```python
from build123d import *

# Parameters (mm, degrees)
SKETCH3_R           = 2.25
SKETCH3_W           = 78.47813411
SKETCH3_H           = 26
BOSS_EXTRUDE1_DEPTH = 3
SKETCH4_W           = 86.47813411
SKETCH4_H           = 3
BOSS_EXTRUDE2_DEPTH = 10


with BuildPart() as part:
    # Sketch3 → Boss-Extrude1 (new body)
    with BuildSketch(Plane(origin=(0, 0, 0), x_dir=(1, 0, 0), z_dir=(0, 1, 0))):
        Polygon((-43.239067055, -30), (-43.239067055, 30), (-39.239067055, 30), (-39.239067055, 21), (39.239067055, 21), (39.239067055, 30), (43.239067055, 30), (43.239067055, -30), (39.239067055, -30), (39.239067055, -21), (-39.239067055, -21), (-39.239067055, -30), align=None)
        with Locations(Location((-26.009067055, 17, 0), (0, 0, 270))):
            Circle(SKETCH3_R, mode=Mode.SUBTRACT)
        with Locations(Location((3.760932945, 16.578763023, 0), (0, 0, 270))):
            Circle(SKETCH3_R, mode=Mode.SUBTRACT)
        with Locations(Location((26.009067055, 17, 0), (0, 0, 270))):
            Circle(SKETCH3_R, mode=Mode.SUBTRACT)
        with Locations(Location((26.009067055, -17, 0), (0, 0, 90))):
            Circle(SKETCH3_R, mode=Mode.SUBTRACT)
        with Locations(Location((3.760932945, -16.578763023, 0), (0, 0, 90))):
            Circle(SKETCH3_R, mode=Mode.SUBTRACT)
        with Locations(Location((-26.009067055, -17, 0), (0, 0, 90))):
            Circle(SKETCH3_R, mode=Mode.SUBTRACT)
        Rectangle(SKETCH3_W, SKETCH3_H, mode=Mode.SUBTRACT)
    extrude(amount=BOSS_EXTRUDE1_DEPTH)

    # Sketch4 → Boss-Extrude2 (add)
    with BuildSketch(Plane.XY.offset(30)):
        with Locations((0, 1.5)):
            Rectangle(SKETCH4_W, SKETCH4_H)
    extrude(amount=BOSS_EXTRUDE2_DEPTH)


solid = part.part
```
Source: CAD feature listing. Evaluate the final solid. Frame: model axes, mm. A direction names the side the tool comes from. Round coordinates to 2 decimals unless told otherwise and drop trailing zeros. Write each loop counter-clockwise with the first axis right and the second up, starting at its lowest first coordinate (ties: lowest second). Pieces come first, ordered by that corner, then holes. Notation, with made-up numbers: M 81,10.5 L 113,10.5 A24 ccw 113,27.5 Z; hole C -15.5,0 d2. An arc over 180 degrees is marked long. Answer as a JSON object with one key per item and string values. Group by question number.
(1) Section query B-B on z = -12. Output: boundary loops of the cut face in (x, y), then the cut area to 3 significant figures.
(2) Section query C-C on y = 1.25. State how many separate pieces and enclosed holes the cut face has, then the cut area to 4 significant figures.
(3) First-contact query: pin 1 (1.5 mm diameter, centred on x = -3.5, y = 1.5, fed in from -Z). Flat tip, straight axial feed; report the tip coordinate or a pass-through.
(4) Ray query, line 1 (Z direction, x = 29, y = 2.05); line 2 (X direction, y = 0.7, z = 0.5); line 3 (X direction, y = 1.8, z = 17). Return the intervals inside material, ascending. Write a range as [from, to].
(5) Section query A-A on x = -2. Output: boundary loops of the cut face in (y, z), then the cut area to 3 significant figures.
(6) Mould query, pull axis Z, two halves, no side actions, for faces 1 (the flat face through (0, 3, 20)), 2 (the flat face through (41, 1, -30)), 3 (the flat face through (-39.239, 1, 0)). Classes: +Z half, -Z half, draft (parallel to the pull), parting line (faces both ways), or undercut.
(7) Reachability of faces 4 (the flat face through (43.239, 1, 5)), 5 (the flat face through (-1, 1, 13)), 6 (the flat face through (-39.239, 1, -26)) from +Z, -Z, +X, -X, +Y, -Y: full face, straight path, thin tool, end or side. Return the list, or none.
Computed values:
{
 "1": {"outline": "M -43.24,0 L -39.24,0 L -39.24,3 L -43.24,3 Z; M 39.24,0 L 43.24,0 L 43.24,3 L 39.24,3 Z", "area": "24.0 mm^2"},
 "2": {"separate pieces": "1", "enclosed holes": "8", "area": "2,505 mm^2"},
 "3": {"pin 1": "z = -21"},
 "4": {"line 1": "[-21, -13], [13, 21], [30, 40]", "line 2": "[-43.24, -39.24], [39.24, 43.24]", "line 3": "[-43.24, -28.26], [-23.76, 1.55], [5.97, 23.76], [28.26, 43.24]"},
 "5": {"outline": "M 0,-21 L 3,-21 L 3,-13 L 0,-13 Z; M 0,13 L 3,13 L 3,21 L 0,21 Z; M 0,30 L 3,30 L 3,40 L 0,40 Z", "area": "78.0 mm^2"},
 "6": {"face 1": "draft", "face 2": "-Z half", "face 3": "undercut"},
 "7": {"face 4": "+Z, -Z, +X, +Y, -Y", "face 5": "+Y, -Y", "face 6": "-Z, +Y, -Y"}
}
